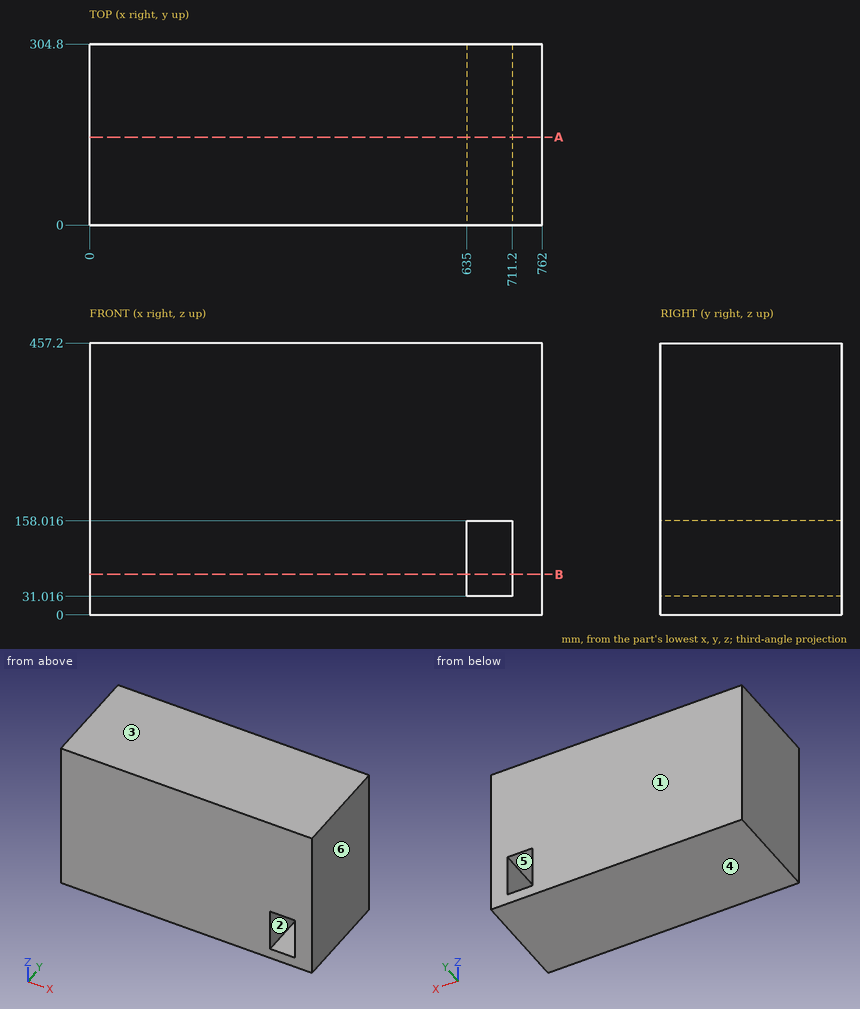
Part print with two shaded views. Sizes in mm from the minimum x, y, z corner. A direction names the side the tool comes from. Coordinates: 2 decimals unless noted, no trailing zeros. Write each loop counter-clockwise with the first axis right and the second up, starting at its lowest first coordinate (ties: lowest second). Pieces come first, ordered by that corner, then holes. Notation, with made-up numbers: (10, 48.5) -> (32, 48.5) arc R13 ccw to (32, 58.5) -> close; hole circle Ø3 at (50, 67.25). An arc over 180 degrees is marked (long way). Return JSON: item names as keys, results as strings. Group by question number.
Q1. Cut at B-B, the plane z = 68. Give the cut face in (x, y), then the cut area to 3 significant figures.
Q2. Flat gauge pin, fed straight in: pin 1 (1.5 mm diameter, centred on y = 87, z = 130.5, fed in from -X). Where does the tip first touch, or does it go through?
Q3. Cut at A-A, the plane y = 148. Give the cut face in (x, z).
Q4. Which spindle directions (+Z, -Z, +X, -X, +Y, -Y) get a long thin tool onto all of the face, cutting with end or side? Do the marked faces 1 and 2. Say none if no direction does.
Q5. Pull direction Z, two halves, no side cores. Call the marked faces 3, 4, 5 and 6: released by +Z, released by -Z, zero draft, split by the parting line, or undercut.
Q6. Drill centre lines: line 1 (X direction, y = 67, z = 40.5); line 2 (Z direction, x = 641, y = 120). Where is each one in solid material? Low to high.
Returned:
{
 "1": {"outline": "(0, 0) -> (635, 0) -> (635, 304.8) -> (0, 304.8) -> close; (711.2, 0) -> (762, 0) -> (762, 304.8) -> (711.2, 304.8) -> close", "area": "209,000 mm2"},
 "2": {"pin 1": "stops at x = 0"},
 "3": {"outline": "(0, 0) -> (762, 0) -> (762, 457.2) -> (0, 457.2) -> close; hole (635, 31.02) -> (711.2, 31.02) -> (711.2, 158.02) -> (635, 158.02) -> close"},
 "4": {"face 1": "+Z, -Z, +X, -X, +Y", "face 2": "+Y, -Y"},
 "5": {"face 3": "released by +Z", "face 4": "released by -Z", "face 5": "undercut", "face 6": "zero draft"},
 "6": {"line 1": "x = 0 to 635, 711.2 to 762", "line 2": "z = 0 to 31.02, 158.02 to 457.2"}
}
